Part model, mm, in its own coordinate system. A direction names the side the tool comes from. Round coordinates to 2 decimals unless told otherwise and drop trailing zeros. Loops run counter-clockwise (first coordinate to the right, second up) from the corner with the lowest first, then second, coordinate; pieces in that order, holes last. Notation, with made-up numbers: M -7.75,60.25 L 14.25,60.25 A18 ccw 14.25,64.25 Z; hole C -4,27.5 d8. An arc over 180 degrees is marked long. Put each result on its own line as item: value. Start each with the question number.
1) Slice it at B-B on z = 11.5. Give the cut face in (x, y), then the cut area to 3 significant figures.
2) Slice it at C-C on x = 55.5. Give the cut face in (y, z), then the cut area to 3 significant figures.
3) Pull direction Z, two halves, no side cores. Call faces 5 (the flat face through (-2.87, -27.3, 39.76)), 6 (the cylindrical face through (2.87, -63.027, 49.942)), 7 (the flat face through (205, -93, 36)): +Z half, -Z half, draft (parallel to the pull), parting line (faces both ways), or undercut.
4) Drop a flat-ended pin along its axis: pin 1 Ø10 at (x, y) = (-51, -27.5) entering from +Z. Give the stop position or say it passes through.
5) Which spindle directions (+Z, -Z, +X, -X, +Y, -Y) get a long thin tool onto all of the face, cutting with end or side? Do faces 1 (the cylindrical face through (100.019, -24.475, 9.86)), 2 (the flat face through (-2.87, -87.65, 78.85)), 3 (the cylindrical face through (2.87, -14.43, 48.48)), 4 (the flat face through (-2.87, -90.08, 73.87)). Say none if no direction does.
6) Slice it at A-A on x = -116. Give the cut face in (y, z), then the cut area to 3 significant figures.
7) Probe line 1 along X through (y, z) = (-30, 7.5); line 2 along Y through (x, z) = (-65, 80); line 3 along Y through (x, z) = (88, 36). List the from-to ranges inside material, lowest first.
```python
from build123d import *

# Parameters (mm, degrees)
F1_DEPTH = 205
F2_R     = 2
F4_DEPTH = 20
F6_DEPTH = 410.001


with BuildPart() as f1:
    # F0 (on Right) → F1 (new body, symmetric)
    with BuildSketch(Plane.YZ):
        with BuildLine():
            Line((-150, 0), (0, 0))
            Line((0, 0), (0, 60.8452405258))
            ThreePointArc((0, 60.8452405258), (-52.9110350074, 45.069498111), (-85, 90))
            Line((-85, 90), (-150, 90))
            Line((-150, 90), (-150, 0))
        make_face()
    extrude(amount=F1_DEPTH, both=True)

    # F2
    f2_edges = [f1.edges().sort_by_distance(p)[0] for p in [
        (0, 0, 60.845241),
    ]]
    fillet(f2_edges, radius=F2_R)

    # F3 (on face) → F4 (cut)
    with BuildSketch(Plane(origin=(0, 0, 0), x_dir=(1, 0, 0), z_dir=(0, 0, -1))):
        with BuildLine():
            ThreePointArc((110, 0), (99.7487373415, 24.7487373415), (75, 35))
            Line((75, 35), (-75, 35))
            ThreePointArc((-75, 35), (-99.7487373415, 24.7487373415), (-110, 0))
            Line((-110, 0), (110, 0))
        make_face()
        with BuildLine():
            ThreePointArc((75, -35), (99.7487373415, -24.7487373415), (110, 0))
            Line((110, 0), (-110, 0))
            ThreePointArc((-110, 0), (-99.7487373415, -24.7487373415), (-75, -35))
            Line((-75, -35), (75, -35))
        make_face()
    extrude(amount=-F4_DEPTH, mode=Mode.SUBTRACT)

    # F5 (on face) → F6 (cut, through all)
    with BuildSketch(Plane(origin=(-205, 0, 0), x_dir=(0, -1, 0), z_dir=(-1, 0, 0))):
        with BuildLine():
            ThreePointArc((35.701952676, 42.5340435067), (31.7112061883, 42.854057797), (27.7615834628, 43.508998254))
            Line((27.7615834628, 43.508998254), (26.8270015062, 35.8974390333))
            Line((26.8270015062, 35.8974390333), (34.7673707193, 34.9224842861))
            Line((34.7673707193, 34.9224842861), (35.701952676, 42.5340435067))
        make_face()
        with BuildLine():
            ThreePointArc((81.5936406798, 72.336454161), (82.9244759082, 76.1123440257), (83.9326143175, 79.9868922087))
            Line((83.9326143175, 79.9868922087), (78.6335187107, 81.6069883197))
            Line((78.6335187107, 81.6069883197), (76.294545073, 73.956550272))
            Line((76.294545073, 73.956550272), (81.5936406798, 72.336454161))
        make_face()
        with BuildLine():
            Line((91.2662483969, 77.7447752641), (83.9326143175, 79.9868922087))
            ThreePointArc((83.9326143175, 79.9868922087), (82.9244759082, 76.1123440257), (81.5936406798, 72.336454161))
            Line((81.5936406798, 72.336454161), (88.9272747591, 70.0943372164))
            Line((88.9272747591, 70.0943372164), (91.2662483969, 77.7447752641))
        make_face()
    extrude(amount=-F6_DEPTH, mode=Mode.SUBTRACT)


solid = f1.part
```
Recorded:
1. outline: M -205,-150 L 205,-150 L 205,0 L 110,0 A35 cw 75,-35 L -75,-35 A35 cw -110,0 L -205,0 Z
1. area: 54,300 mm2
2. outline: M -150,0 L -35,0 L -35,20 L 0,20 L 0,55.5 A2 ccw -3.43,56.9 A47.5 cw -27.76,43.51 L -26.83,35.9 L -34.77,34.92 L -35.7,42.53 A47.5 cw -81.59,72.34 L -88.93,70.09 L -91.27,77.74 L -83.93,79.99 A47.5 cw -85,90 L -150,90 Z
2. area: 9,330 mm2
3. face 5: undercut
3. face 6: +Z half
3. face 7: draft
4. pin 1: stops at z = 44.93
5. face 1: -Z, +Y
5. face 2: +X, -X, +Y
5. face 3: +Z, +X, -X
5. face 4: +X, -X
6. outline: M -150,0 L 0,0 L 0,55.5 A2 ccw -3.43,56.9 A47.5 cw -27.76,43.51 L -26.83,35.9 L -34.77,34.92 L -35.7,42.53 A47.5 cw -81.59,72.34 L -88.93,70.09 L -91.27,77.74 L -83.93,79.99 A47.5 cw -85,90 L -150,90 Z
6. area: 10,000 mm2
7. line 1: x = -205 to -93.03, 93.03 to 205
7. line 2: y = -150 to -83.94
7. line 3: y = -150 to -34.9, -26.84 to 0
